```python
from build123d import *

# Parameters (mm, degrees)
FILLET_1_R               = 4
CUT_EXTRUDE_10_DEPTH     = 201
PATTERN_CIRCULAR_1_COUNT = 6
FILLET_2_R               = 5
SKETCH_10_W              = 6.3
SKETCH_10_H              = 8
CUT_EXTRUDE_13_DEPTH     = 201
SKETCH_11_R              = 6.62185
CUT_EXTRUDE_14_DEPTH     = 201
SKETCH_12_R              = 6
CUT_EXTRUDE_15_DEPTH     = 201


with BuildPart() as part:
    # Sketch 1 → Revolve 1 (revolve)
    with BuildSketch(Plane(origin=(0, 0, 0), x_dir=(1, 0, 0), z_dir=(0, 1, 0)), mode=Mode.PRIVATE) as revolve_1_sk:
        Polygon((15, 20), (30, 20), (30, 6), (70, 6), (70, 15), (100, 15), (100, -15), (70, -15), (70, -6), (30, -6), (30, -20), (15, -20), align=None)
    revolve(revolve_1_sk.sketch.rotate(Axis((0, 0, -20), (0, 0, 1)), 180), axis=Axis((0, 0, -20), (0, 0, 1)))

    # Fillet 1
    fillet_1_edges = [part.edges().sort_by_distance(p)[0] for p in [
        (70, 0, 15),
        (70, 0, -15),
        (30, 0, -20),
        (30, 0, 20),
    ]]
    fillet(fillet_1_edges, radius=FILLET_1_R)

    # Sketch 8 → Cut-Extrude 10 (cut, symmetric)
    with BuildSketch(Plane.XY):
        with BuildLine():
            Line((37.5233, 6), (61.709, 6))
            ThreePointArc((61.709, 6), (53.693260927, 30.999195997), (36.0505, 50.44))
            Line((36.0505, 50.44), (23.9577, 29.4952))
            ThreePointArc((23.9577, 29.4952), (32.908424465, 18.999310823), (37.5233, 6))
        make_face()
    cut_extrude_10 = extrude(amount=CUT_EXTRUDE_10_DEPTH, both=True, mode=Mode.SUBTRACT)

    # Pattern Circular 1: Cut-Extrude 10 ×6 about axis
    pattern_circular_1_axis = Axis((0, 0, 0), (0, 0, 1))
    for i in range(1, PATTERN_CIRCULAR_1_COUNT):
        add(cut_extrude_10.rotate(pattern_circular_1_axis, i * 360 / PATTERN_CIRCULAR_1_COUNT), mode=Mode.SUBTRACT)

    # Fillet 2
    fillet_2_edges = [part.edges().sort_by_distance(p)[0] for p in [
        (-37.5233, -6, 0),
        (-23.9577, -29.4952, 0),
        (-36.0505, -50.44, 0),
        (-61.709, -6, 0),
        (-23.957802423, 29.496131034, 0),
        (-37.52244249, 6.000376816, 0),
        (-61.707571367, 6.000648819, 0),
        (-36.050652423, 50.441561642, 0),
        (13.565497577, 35.496131034, 0),
        (-13.56474249, 35.495576816, 0),
        (-25.657071367, 56.440648819, 0),
        (25.658347577, 56.441561642, 0),
        (37.5233, 6, 0),
        (23.9577, 29.4952, 0),
        (36.0505, 50.44, 0),
        (61.709, 6, 0),
        (23.957802423, -29.496131034, 0),
        (37.52244249, -6.000376816, 0),
        (61.707571367, -6.000648819, 0),
        (36.050652423, -50.441561642, 0),
        (-13.565497577, -35.496131034, 0),
        (13.56474249, -35.495576816, 0),
        (25.657071367, -56.440648819, 0),
        (-25.658347577, -56.441561642, 0),
    ]]
    fillet(fillet_2_edges, radius=FILLET_2_R)

    # Sketch 10 → Cut-Extrude 13 (cut, symmetric)
    with BuildSketch(Plane.XY):
        with Locations((15.15, 0)):
            Rectangle(SKETCH_10_W, SKETCH_10_H)
    extrude(amount=CUT_EXTRUDE_13_DEPTH, both=True, mode=Mode.SUBTRACT)

    # Sketch 11 → Cut-Extrude 14 (cut, symmetric)
    with BuildSketch(Plane.XY):
        with Locations(Location((-80, 0, 0), (0, 0, 335.993504464))):
            Circle(SKETCH_11_R)
    extrude(amount=CUT_EXTRUDE_14_DEPTH, both=True, mode=Mode.SUBTRACT)

    # Sketch 12 → Cut-Extrude 15 (cut, symmetric)
    with BuildSketch(Plane.XY):
        with Locations((92, 0)):
            Circle(SKETCH_12_R)
    extrude(amount=CUT_EXTRUDE_15_DEPTH, both=True, mode=Mode.SUBTRACT)


solid = part.part
```
Geometry check sheet. Reference: the model listing, model coordinates, mm. A direction names the side the tool comes from. Round coordinates to 2 decimals unless told otherwise and drop trailing zeros. Order: outer loops, then holes, each group sorted by start corner. A loop starts at its lowest first (then second) coordinate and runs counter-clockwise, first axis right, second up. Notation, with made-up numbers: (72, 73) - (120, 73) arc R24 cw to (120, 103) - close; hole circle Ø11 at (4, 68.25). An arc over 180 degrees is marked (long way). Use a Markdown table: item, result. Add a question column.
(1) Release check for a two-part mould opening along Y. For faces 3 (the flat face through (11, 11, -20)), 4 (the cylindrical face through (13.207, 36.895, -0.084)) record: pulls with the +Y half, pulls with the -Y half, needs draft (parallel to the pull), parting line crosses it, or undercut.
(2) Depth check by flat-ended pin: pin 1 (4 mm diameter, centred on y = -78.5, z = -9.5, fed in from +X); pin 2 (3 mm diameter, centred on x = 17, z = 7.5, fed in from +Y); pin 3 (1.5 mm diameter, centred on x = -70.5, z = 5, fed in from -Y). Enter the tip coordinate at first touch or a pass-through.
(3) Sectioned sample at D-D, the plane x = 92. Enter the section's corners in (y, z), and give its area (3 significant figures).
(4) Material ranges on line 1 along Y through (x, z) = (0, -2.5); line 2 along Y through (x, z) = (7, 0); line 3 along X through (y, z) = (27, 1.5), recorded low to high. Write a range as [from, to].
(5) Sectioned sample at B-B, the plane x = 0. Count the separate pieces of the cut face and the enclosed holes in it, and give its area (3 significant figures).
(6) Sectioned sample at A-A, the plane x = -80. Enter the section's corners in (y, z).
(7) Tool access check on faces 1 (the cylindrical face through (-32.84, -19.12, 0.08)), 2 (the flat face through (-30, 15, 6)). Record the directions out of +Z, -Z, +X, -X, +Y, -Y that give a thin tool (end or side, any length) a straight path to the whole face; none if there is none.
Answers below:
| question | item | result |
|---|---|---|
| 1 | face 3 | needs draft |
| 1 | face 4 | undercut |
| 2 | pin 1 | x = 64.4 |
| 2 | pin 2 | y = 98.79 |
| 2 | pin 3 | y = -71.66 |
| 3 | outline | (-39.19, -15) - (-6, -15) - (-6, 15) - (-39.19, 15) - close; (6, -15) - (39.19, -15) - (39.19, 15) - (6, 15) - close |
| 3 | area | 1,990 mm² |
| 4 | line 1 | [-100, -62], [-38, -15], [15, 38], [62, 100] |
| 4 | line 2 | [-99.75, -61.6], [-37.35, -13.27], [13.27, 37.35], [61.6, 99.75] |
| 4 | line 3 | [-96.29, -55.81], [-26.74, 26.74], [55.81, 96.29] |
| 5 | separate pieces | 4 |
| 5 | enclosed holes | 0 |
| 5 | area | 3,360 mm² |
| 6 | outline | (-60, -15) - (-6.62, -15) - (-6.62, 15) - (-60, 15) - close; (6.62, -15) - (60, -15) - (60, 15) - (6.62, 15) - close |
| 7 | face 1 | +Z, -Z |
| 7 | face 2 | +Z |
